Could you check a few things on this model? Use its own coordinates, in mm. Give positions to 0.01 mm unless a question says otherwise; leave off trailing zeros. Order: outer loops, then holes, each group sorted by start corner. A loop starts at its lowest first (then second) coordinate and runs counter-clockwise, first axis right, second up.
from build123d import *

# Parameters (mm, degrees)
F0_W     = 54.3647520244
F0_H     = 52.432758268
F2_DEPTH = 325.374
F1_W     = 125.3076829016
F1_H     = 105.2813343704
F1_W_2   = 63.1306562573
F1_H_2   = 22.8872485459
F1_R     = 36.1337810963
F3_DEPTH = 232.156


with BuildPart() as f2:
    # F0 (on Front) → F2 (new body)
    with BuildSketch(Plane.XZ):
        with Locations((-82.3284629732, 22.3198619206)):
            Rectangle(F0_W, F0_H)
    extrude(amount=F2_DEPTH)

    # F1 (on Top) → F3 (join)
    with BuildSketch(Plane.XY):
        with Locations((2.4547781795, -13.0648035556)):
            Rectangle(F1_W, F1_H)
        with Locations((1.3104146346, -50.0658545643)):
            Rectangle(F1_W_2, F1_H_2, mode=Mode.SUBTRACT)
        Circle(F1_R, mode=Mode.SUBTRACT)
        Circle(F1_R)
    extrude(amount=F3_DEPTH)


solid = f2.part
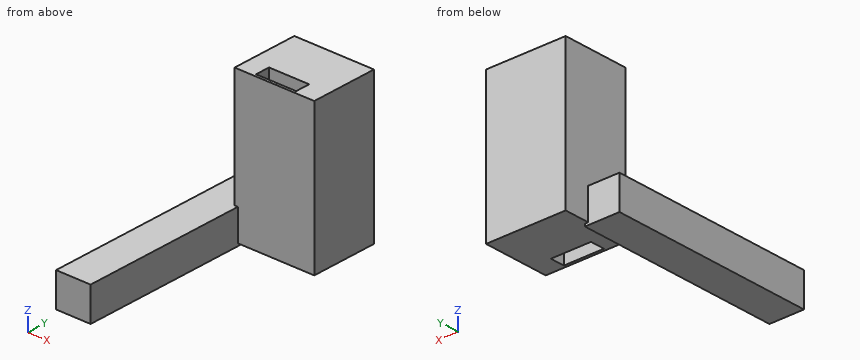
Item 1: Please list where these lines run through material, in increasing order: line 1 along Y through (x, z) = (-9.5, 200); line 2 along Z through (x, y) = (-60.5, -157); line 3 along X through (y, z) = (-92, 6).
Findings:
line 1: y = -65.71 to -61.51, -38.62 to 39.58
line 2: z = -3.9 to 48.54
line 3: x = -109.51 to -55.15
Item 2: Imagine slicing it at A-A on x = -12. List the corners of the cut face in (y, z) for me.
Findings:
outline: (-65.71, 0) - (-61.51, 0) - (-61.51, 232.16) - (-65.71, 232.16) - close; (-38.62, 0) - (39.58, 0) - (39.58, 232.16) - (-38.62, 232.16) - close
Item 3: Imagine slicing it at C-C on z = 15. List the corners of the cut face in (x, y) for me, then the cut area to 3 significant figures.
Findings:
outline: (-109.51, -325.37) - (-55.15, -325.37) - (-55.15, -65.71) - (65.11, -65.71) - (65.11, 39.58) - (-60.2, 39.58) - (-60.2, 0) - (-109.51, 0) - close; hole (-30.25, -61.51) - (32.88, -61.51) - (32.88, -38.62) - (-30.25, -38.62) - close
area: 29,100 mm2
Item 4: Imagine slicing it at D-D on x = -95.5. List the corners of the cut face in (y, z) for me.
Findings:
outline: (-325.37, -3.9) - (0, -3.9) - (0, 48.54) - (-325.37, 48.54) - close
Item 5: Imagine slicing it at B-B on z = 89. List the corners of the cut face in (x, y) for me, then the cut area to 3 significant figures.
Findings:
outline: (-60.2, -65.71) - (65.11, -65.71) - (65.11, 39.58) - (-60.2, 39.58) - close; hole (-30.25, -61.51) - (32.88, -61.51) - (32.88, -38.62) - (-30.25, -38.62) - close
area: 11,700 mm2
Item 6: For pin 1 (7 mm diameter, centred on y = -53, z = 92.5, fed in from -X), with a flat end and sliding along its axis, tell me the tip position at first contact or that it passes through.
Findings:
pin 1: stops at x = -60.2
